For this review, take the finished solid that the model builds, in its own axes (mm). A direction names the side the tool comes from. Give positions to 0.01 mm unless a question says otherwise; leave off trailing zeros. Order: outer loops, then holes, each group sorted by start corner. A loop starts at its lowest first (then second) coordinate and runs counter-clockwise, first axis right, second up. Notation, with made-up numbers: M 71.5,-14.5 L 127.5,-14.5 A22 ccw 127.5,7.5 Z; hole C -10.5,-10.5 d10. An arc over 180 degrees is marked long. Answer as CSV lines item,"result". Start each with the question number.
1. Clearance check with flat-ended pins moving along their axes: P1, Ø12, axis at y = 19, z = 4, coming from the +X side (3 decimals); P2, Ø4, axis at x = 18.5, z = 54.5, coming from the +Y side; P3, Ø10, axis at y = 19, z = 37, coming from the -X side. State where each tip first meets the part, or that it passes through.
2. Machinability: for faces 1 (the flat face through (41.275, -1, 4)), 2 (the cylindrical face through (32.052, -16.791, 51.286)), 3 (the cylindrical face through (32.052, 16.547, 51.286)), which of the approach directions +Z, -Z, +X, -X, +Y, -Y give a long, thin tool a straight path to every point of the face, cutting with its end or side? Answer none if there is none.
3. We need section C-C, the plane x = 68.5. Give the boundary of the cut face in (y, z).
4. For line 1 along X through (y, z) = (-32.5, 8) (3 decimals); line 2 along Z through (x, y) = (14.5, 33.5) (3 decimals); line 3 along Y through (x, z) = (77, 53), list the stretches that pass through material, from the lowest coordinate up.
5. We need section A-A, the plane z = 2.5. Give the boundary of the cut face in (x, y) (3 decimals), and give its area (3 significant figures).
6. Mouldability with a two-part tool opening along X and no side actions: class faces 4 (the flat face through (66, 0, 42.875)), 5 (the flat face through (80.51, -23, 52)), 6 (the flat face through (0, 63.5, 0)), 7 (the cylindrical face through (39.464, -61.59, 0.133)) as pulls with the +X half, pulls with the -X half, needs draft (parallel to the pull), parting line crosses it, or undercut.
7. We need section B-B, the plane y = 39. Give the boundary of the cut face in (x, z) (3 decimals).
from build123d import *

# Parameters (mm, degrees)
F1_DEPTH = 63.5
F2_DEPTH = 25.4
F3_DEPTH = 7.9375
F5_R     = 6.35


with BuildPart() as f1:
    # F0 (on Front) → F1 (new body, symmetric)
    with BuildSketch(Plane.XZ):
        Polygon((22.225, 9.525), (-41.275, 9.525), (-41.275, -9.525), (41.275, -9.525), (41.275, 9.525), align=None)
    extrude(amount=F1_DEPTH, both=True)

    # F0 (on Front) → F2 (join, symmetric)
    with BuildSketch(Plane.XZ):
        with BuildLine():
            Line((22.225, 27.0002), (22.225, 9.525))
            Line((22.225, 9.525), (41.275, 9.525))
            Line((41.275, 9.525), (41.275, 27.0002))
            ThreePointArc((41.275, 27.0002), (45.9246798487, 38.2255201513), (57.15, 42.8752))
            Line((57.15, 42.8752), (80.509888177, 42.8752))
            Line((80.509888177, 42.8752), (80.509888177, 61.9252))
            Line((80.509888177, 61.9252), (57.15, 61.9252))
            add(Edge.make_bspline(
                [(55.2606607544, 61.8740587228), (55.8984719216, 61.8948615926), (56.5284123731, 61.9118838852), (57.15, 61.9252)],
                knots=[109.5520326142, 109.5520326142, 109.5520326142, 109.5520326142, 111.5045361635, 111.5045361635, 111.5045361635, 111.5045361635], degree=3))
            ThreePointArc((55.2606607544, 61.8740587228), (31.7951109433, 51.0186351265), (22.225, 27.0002))
        make_face()
    extrude(amount=F2_DEPTH, both=True)

    # F0 (on Front) → F3 (join, symmetric)
    with BuildSketch(Plane.XZ):
        with BuildLine():
            add(Edge.make_bspline(
                [(-41.275, 9.525), (-41.0908827839, 47.6377500775), (19.4740370552, 60.7068410375), (55.2606607544, 61.8740587228)],
                knots=[0, 0, 0, 0, 109.5520326142, 109.5520326142, 109.5520326142, 109.5520326142], degree=3))
            Line((-41.275, 9.525), (22.225, 9.525))
            Line((22.225, 9.525), (22.225, 27.0002))
            ThreePointArc((22.225, 27.0002), (31.7951109433, 51.0186351265), (55.2606607544, 61.8740587228))
        make_face()
    extrude(amount=F3_DEPTH, both=True)

    # F0 (on Front) → F4 (revolve)
    with BuildSketch(Plane.XZ):
        Polygon((131.309888177, 66.675), (101.6, 66.675), (101.9684821367, 38.1), (131.309888177, 38.1), align=None)
    revolve(axis=Axis((101.7842410684, 0, 52.3875), (-0.0128941908, 0, 0.9999168665)))

    # F5
    f5_edges = [f1.edges().sort_by_distance(p)[0] for p in [
        (41.275, -63.5, 0),
        (-41.275, -63.5, 0),
        (-41.275, 63.5, 0),
        (41.275, 63.5, 0),
    ]]
    fillet(f5_edges, radius=F5_R)


solid = f1.part
Result set:
1,P1,"x = 41.275"
1,P2,"y = 7.94"
1,P3,"x = 22.58"
2,face 1,"-Z, +X, +Y, -Y"
2,face 2,"+Z, -X, -Y"
2,face 3,"+Z, -X, +Y"
3,outline,"M -25.4,42.88 L 25.4,42.88 L 25.4,61.93 L -25.4,61.93 Z"
4,line 1,"-41.275 to 41.275"
4,line 2,"-9.525 to 9.525"
4,line 3,"-25.4 to 25.4"
5,outline,"M -41.275,-57.15 A6.35 ccw -34.925,-63.5 L 34.925,-63.5 A6.35 ccw 41.275,-57.15 L 41.275,57.15 A6.35 ccw 34.925,63.5 L -34.925,63.5 A6.35 ccw -41.275,57.15 Z"
5,area,"10,400 mm2"
6,face 4,"undercut"
6,face 5,"undercut"
6,face 6,"needs draft"
6,face 7,"pulls with the +X half"
7,outline,"M -41.275,-9.525 L 41.275,-9.525 L 41.275,9.525 L -41.275,9.525 Z"
